```python
from build123d import *

# Parameters (mm, degrees)
SKETCH1_W                       = 45
SKETCH1_H                       = 86
SKETCH1_R                       = 7.1
BOSS_EXTRUDE1_DEPTH             = 4
BOSS_EXTRUDE2_DEPTH             = 45
SKETCH3_W                       = 45
SKETCH3_H                       = 5.372111066
BOSS_EXTRUDE3_DEPTH             = 40
BOSS_EXTRUDE3_DIRECTION_2_REACH = 70.185
SKETCH4_W                       = 45
SKETCH4_H                       = 5.372111066
BOSS_EXTRUDE4_DEPTH             = 3.295
SKETCH5_W                       = 18.57978737
SKETCH5_H                       = 1.409707481
BOSS_EXTRUDE5_DEPTH             = 44.189029
CHAMFER2_SIZE                   = 1.405
BOSS_EXTRUDE7_DEPTH             = 45
SKETCH8_R                       = 1.375
CUT_EXTRUDE1_DEPTH              = 125.392527932
CHAMFER3_SIZE                   = 10
CHAMFER4_SIZE                   = 1.75
SKETCH9_R                       = 11
SKETCH9_W                       = 45
SKETCH9_H                       = 4.475285766
BOSS_EXTRUDE8_DEPTH             = 1.9


with BuildPart() as part:
    # Sketch1 → Boss-Extrude1 (new body)
    with BuildSketch(Plane.XY):
        with Locations((0, -1)):
            Rectangle(SKETCH1_W, SKETCH1_H)
        with Locations((0, 19.65)):
            Circle(SKETCH1_R, mode=Mode.SUBTRACT)
        with Locations((0, -28.15)):
            Circle(SKETCH1_R, mode=Mode.SUBTRACT)
    extrude(amount=BOSS_EXTRUDE1_DEPTH)

    # Sketch2 → Boss-Extrude2 (add)
    with BuildSketch(Plane(origin=(22.5, 0, 0), x_dir=(0, 0, -1), z_dir=(1, 0, 0))):
        with BuildLine():
            Line((-4, 42), (-17.385970531, 56.343405204))
            add(Edge.make_bspline(
                [(-18.399488548, 61.71551627), (-17.964102111, 59.93301782), (-17.698797731, 58.135329436), (-17.385970531, 56.343405204)],
                knots=[0.068292811, 0.068292811, 0.068292811, 0.068292811, 0.115576408, 0.115576408, 0.115576408, 0.115576408], degree=3))
            Line((-18.399488548, 61.71551627), (0, 42))
            Line((0, 42), (-4, 42))
        make_face()
    extrude(amount=-BOSS_EXTRUDE2_DEPTH)

    # Sketch3 → Boss-Extrude3 (add)
    with BuildSketch(Plane.XY.offset(18.28)):
        with Locations((0, 59.029460737)):
            Rectangle(SKETCH3_W, SKETCH3_H)
    extrude(amount=BOSS_EXTRUDE3_DEPTH)

    # Sketch3 → Boss-Extrude3 direction 2 (add, up to next)
    with BuildSketch(Plane.XY.offset(18.28), mode=Mode.PRIVATE) as boss_extrude3_direction_2_sk1:
        with Locations((0, 59.029460737)):
            Rectangle(SKETCH3_W, SKETCH3_H)
    boss_extrude3_direction_2_tool1 = extrude(boss_extrude3_direction_2_sk1.sketch, amount=-BOSS_EXTRUDE3_DIRECTION_2_REACH, mode=Mode.PRIVATE) - part.part
    add(boss_extrude3_direction_2_tool1.solids().sort_by_distance((0, 59.029461, 18.28))[0])

    # Sketch4 → Boss-Extrude4 (add)
    with BuildSketch(Plane.XY.offset(58.28)):
        with Locations((0, 59.029460737)):
            Rectangle(SKETCH4_W, SKETCH4_H)
    extrude(amount=BOSS_EXTRUDE4_DEPTH)

    # Sketch5 → Boss-Extrude5 (add)
    with BuildSketch(Plane.XY.offset(61.575)):
        with Locations((-0.00312038, 55.638551464)):
            Rectangle(SKETCH5_W, SKETCH5_H)
    extrude(amount=-BOSS_EXTRUDE5_DEPTH)

    # Chamfer2
    chamfer2_edges = [part.edges().sort_by_distance(p)[0] for p in [
        (-0.00312038, 54.933697723, 17.385971),
    ]]
    chamfer(chamfer2_edges, length=CHAMFER2_SIZE)

    # Sketch7 → Boss-Extrude7 (add)
    with BuildSketch(Plane(origin=(22.5, 0, 0), x_dir=(0, 0, -1), z_dir=(1, 0, 0))):
        Polygon((-18.28, 61.71551627), (-16.793697174, 61.71551627), (0, 43.720645978), (0, 42), (-18.28, 61.587481275), align=None)
    extrude(amount=-BOSS_EXTRUDE7_DEPTH)

    # Sketch8 → Cut-Extrude1 (cut, through all)
    with BuildSketch(Plane(origin=(0, 61.71551627, 0), x_dir=(1, 0, 0), z_dir=(0, 1, 0))):
        with Locations(Location((15.735, -50.299042534, 0), (0, 0, 180))):
            Circle(SKETCH8_R)
        with Locations(Location((15.735, -34.097127603, 0), (0, 0, 180))):
            Circle(SKETCH8_R)
        with Locations(Location((-15.743014065, -34.097127603, 0), (0, 0, 180))):
            Circle(SKETCH8_R)
        with Locations(Location((-15.743014065, -50.299042534, 0), (0, 0, 180))):
            Circle(SKETCH8_R)
    extrude(amount=-CUT_EXTRUDE1_DEPTH, mode=Mode.SUBTRACT)

    # Chamfer3
    chamfer3_edges = [part.edges().sort_by_distance(p)[0] for p in [
        (22.5, -44, 2),
        (-22.5, -44, 2),
    ]]
    chamfer(chamfer3_edges, length=CHAMFER3_SIZE)

    # Chamfer4
    chamfer4_edges = [part.edges().sort_by_distance(p)[0] for p in [
        (22.5, 4.860322989, 0),
        (0, -44, 0),
        (-17.5, -39, 0),
        (17.5, -39, 0),
        (-22.5, 4.860322989, 0),
    ]]
    chamfer(chamfer4_edges, length=CHAMFER4_SIZE)

    # Sketch9 → Boss-Extrude8 (add)
    # profile 1 of 2: a face of its own
    with BuildSketch(Plane.XY.offset(4)):
        Polygon((-22.5, -34), (-12.5, -44), (12.5, -44), (22.5, -34), (22.5, 42), (-22.5, 42), align=None)
        with Locations(Location((0, -28.15, 0), (0, 0, 180))):
            Circle(SKETCH9_R, mode=Mode.SUBTRACT)
        with Locations(Location((0, 19.65, 0), (0, 0, 180))):
            Circle(SKETCH9_R, mode=Mode.SUBTRACT)
    # profile 2 of 2: a face of its own
    with BuildSketch(Plane.XY.offset(4)):
        with Locations((0, 44.237642883)):
            Rectangle(SKETCH9_W, SKETCH9_H)
    extrude(amount=BOSS_EXTRUDE8_DEPTH)


solid = part.part
```
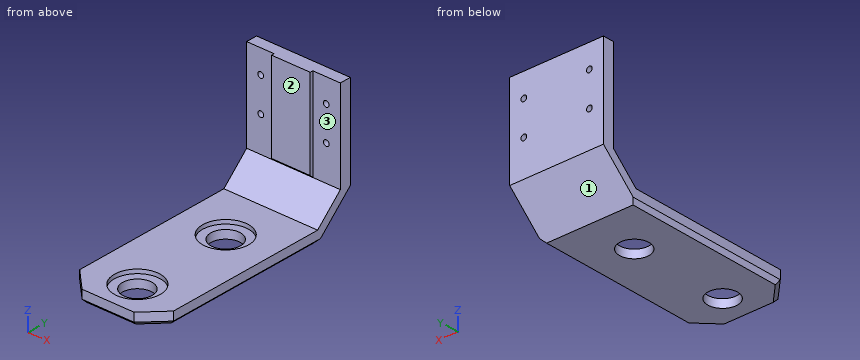
Geometry: final body of the model. Coordinates: model frame, mm. Face numbers are marked on the shaded views. A direction names the side the tool comes from. Round coordinates to 2 decimals unless told otherwise and drop trailing zeros. Order: outer loops, then holes, each group sorted by start corner. A loop starts at its lowest first (then second) coordinate and runs counter-clockwise, first axis right, second up. Notation, with made-up numbers: (62.5, 10.25) -> (83.5, 10.25) arc R24 cw to (83.5, 44.25) -> close; hole circle Ø1 at (8.5, 46). An arc over 180 degrees is marked (long way). Use CSV: the item, a comma, the result in double quotes. Start each with the question number.
1) Material intervals for line 1 along Z through (x, y) = (-19, 27.5); line 2 along Z through (x, y) = (6.5, -24.5); line 3 along Y through (x, z) = (0, 51), sorted ascending. Write a range as from..to.
2) First-contact query: pin 1 Ø8 at (x, z) = (-9, 44) entering from -Y; pin 2 Ø6.5 at (x, y) = (1, 14.5) entering from +Z; pin 3 Ø3 at (x, y) = (-0.5, 33) entering from +Z. Flat tips, straight axial feed; report the tip coordinate or a pass-through.
3) Section C-C (x = 0). Return the cut outline in (y, z) (3 decimals).
4) Set-up query: the marked faces 1, 2 and 3. Return all of +Z, -Z, +X, -X, +Y, -Y with unobstructed straight access to the full face (end or side cutting, diameter ignored); none if empty.
5) Section B-B (z = 53). Return the cut outline in (x, y), and give its area (3 significant figures).
6) Section A-A (y = 19.65). Return the cut outline in (x, z), and give its area (3 significant figures).
7) Section D-D (y = 4). Return the cut outline in (x, z), and give its area (3 significant figures).
Returned:
1,line 1,"z = 0..5.9"
1,line 2,"z = 0..4"
1,line 3,"y = 54.93..61.72"
2,pin 1,"stops at y = 54.93"
2,pin 2,"stops at z = 4"
2,pin 3,"stops at z = 5.9"
3,outline,"(-44, 1.75) -> (-42.25, 0) -> (-35.25, 0) -> (-35.25, 4) -> (-39.15, 4) -> (-39.15, 5.9) -> (-44, 5.9) -> close; (-21.05, 0) -> (12.55, 0) -> (12.55, 4) -> (8.65, 4) -> (8.65, 5.9) -> (-17.15, 5.9) -> (-17.15, 4) -> (-21.05, 4) -> close; (26.75, 0) -> (43.721, 0) -> (61.716, 16.794) -> (61.716, 61.575) -> (54.934, 61.575) -> (54.934, 18.791) -> (56.339, 17.386) -> (56.343, 17.386) -> (44.036, 5.9) -> (30.65, 5.9) -> (30.65, 4) -> (26.75, 4) -> close"
4,face 1,"-Z, +X, -X, +Y"
4,face 2,"+Z, +X, -X, -Y"
4,face 3,"+Z, +X, -Y"
5,outline,"(-22.5, 56.34) -> (-9.29, 56.34) -> (-9.29, 54.93) -> (9.29, 54.93) -> (9.29, 56.34) -> (22.5, 56.34) -> (22.5, 61.72) -> (-22.5, 61.72) -> close"
5,area,"268 mm²"
6,outline,"(-22.5, 1.75) -> (-20.75, 0) -> (-7.1, 0) -> (-7.1, 4) -> (-11, 4) -> (-11, 5.9) -> (-22.5, 5.9) -> close; (7.1, 0) -> (20.75, 0) -> (22.5, 1.75) -> (22.5, 5.9) -> (11, 5.9) -> (11, 4) -> (7.1, 4) -> close"
6,area,"164 mm²"
7,outline,"(-22.5, 1.75) -> (-20.75, 0) -> (20.75, 0) -> (22.5, 1.75) -> (22.5, 5.9) -> (-22.5, 5.9) -> close"
7,area,"262 mm²"
